Build history of the part. All positions in model axes, mm. A direction names the side the tool comes from. Give positions to 0.01 mm unless a question says otherwise; leave off trailing zeros. Order: outer loops, then holes, each group sorted by start corner. A loop starts at its lowest first (then second) coordinate and runs counter-clockwise, first axis right, second up. Notation, with made-up numbers: M 71,-14 L 106,-14 A23 cw 106,21 Z; hole C -28.75,41.5 d9. An arc over 180 degrees is marked long. Use CSV: the item, a comma, the result in double quotes. Start each with the question number.
Item 1: Which spindle directions (+Z, -Z, +X, -X, +Y, -Y) get a long thin tool onto all of the face, cutting with end or side? Do faces 5 (the flat face through (7, 17, -36.065)), 6 (the flat face through (9, -55.144, 26)), 7 (the flat face through (17, -53.044, 26)). Say none if no direction does.
Item 2: Wall check: line 1 along Z through (x, y) = (11.5, 75); line 2 along Z through (x, y) = (18, -24.5); line 3 along Y through (x, z) = (9.5, 3). Give the ranges that are in metal, low to high.
Item 3: Band-saw the part on A-A on y = 71.5. Write the cut outline in (x, z), plus the area to 3 significant figures.
Item 4: Two-plate mould, pull along Z, no slides. Class faces 1 (the flat face through (9, 90.856, 26)), 2 (the flat face through (9, 17, -46.065)), 3 (the flat face through (9, 17, 99.935)), 4 (the flat face through (7, 17, 89.935)): pulls with the +Z half, pulls with the -Z half, needs draft (parallel to the pull), parting line crosses it, or undercut.
Item 5: Band-saw the part on B-B on x = 6.5. Write the cut outline in (y, z), plus the area to 3 significant figures.
Item 6: Band-saw the part on C-C on z = 53.5. Write the cut outline in (x, y).
from build123d import *

# Parameters (mm, degrees)
F0_W     = 146
F0_H     = 146
F1_DEPTH = 19
F2_W     = 126
F2_H     = 126
F3_DEPTH = 25
F4_W     = 141.8
F4_H     = 141.8
F5_DEPTH = 5


# Not quite as in the source:
# - a feature names something its author has since deleted; it is built from what else it names


with BuildPart() as f1:
    # F0 (on Right) → F1 (new body)
    with BuildSketch(Plane.YZ):
        with Locations((17.8558837175, 26.935071826)):
            Rectangle(F0_W, F0_H)
    extrude(amount=F1_DEPTH)

    # F2 (on face) → F3 (cut)
    with BuildSketch(Plane.YZ.offset(19)):
        with Locations((17.8558837175, 26.935071826)):
            Rectangle(F2_W, F2_H)
    extrude(amount=-F3_DEPTH, mode=Mode.SUBTRACT)

    # F4 (on face) → F5 (cut)
    with BuildSketch(Plane.YZ.offset(19)):
        with Locations((17.8558837175, 26.935071826)):
            Rectangle(F4_W, F4_H)
    extrude(amount=-F5_DEPTH, mode=Mode.SUBTRACT)


solid = f1.part
Model answer:
1,face 5,"+X, -X"
1,face 6,"+Z, -Z, +X, -X, -Y"
1,face 7,"+X"
2,line 1,"z = -46.06 to -36.06, 89.94 to 99.94"
2,line 2,"z = -46.06 to -43.96, 97.84 to 99.94"
2,line 3,"y = -55.14 to -45.14, 80.86 to 90.86"
3,outline,"M 0,-46.06 L 19,-46.06 L 19,-43.96 L 14,-43.96 L 14,-36.06 L 0,-36.06 Z; M 0,89.94 L 14,89.94 L 14,97.84 L 19,97.84 L 19,99.94 L 0,99.94 Z"
3,area,"301 mm^2"
4,face 1,"needs draft"
4,face 2,"pulls with the -Z half"
4,face 3,"pulls with the +Z half"
4,face 4,"undercut"
5,outline,"M -55.14,-46.06 L 90.86,-46.06 L 90.86,99.94 L -55.14,99.94 Z; hole M -45.14,-36.06 L 80.86,-36.06 L 80.86,89.94 L -45.14,89.94 Z"
5,area,"5,440 mm^2"
6,outline,"M 0,-55.14 L 19,-55.14 L 19,-53.04 L 14,-53.04 L 14,-45.14 L 0,-45.14 Z; M 0,80.86 L 14,80.86 L 14,88.76 L 19,88.76 L 19,90.86 L 0,90.86 Z"
